The listing builds one solid part. Answer for the finished solid, in the listing's coordinates (mm). Round coordinates to 2 decimals unless told otherwise and drop trailing zeros. Loops run counter-clockwise (first coordinate to the right, second up) from the corner with the lowest first, then second, coordinate; pieces in that order, holes last. Notation, with made-up numbers: M 36,-22.5 L 55,-22.5 A8 cw 55,-16.5 Z; hole C 88,-40 d6. An arc over 180 degrees is marked long. Put each result on its own line as item: value. Start each with the question number.
(1) Straight lines are drawn through the part: line 1 (X direction, y = -20.75, z = 104.9); line 2 (Y direction, x = -20, z = 104.85); line 3 (Y direction, x = 0.5, z = 104.65). For each, find the intervals that lie inside material, in ascending order.
(2) Section C-C, the plane x = 0 is taken. Determine the outline of the cut face in (y, z), then the cut area to 3 significant figures.
(3) Section A-A, the plane z = 104.1 is taken. Determine the outline of the cut face in (x, y).
(4) Determine the mould class of faces 1 (the face through (8, -14, 105.1)), 2 (the face through (0, -8, 104)), 3 (the face through (-1.5, -11.1, 104.4)) for opening direction X: released by +X, released by -X, zero draft, split by the parting line, or undercut.
(5) Section B-B, the plane y = -22.5 is taken. Determine the outline of the cut face in (x, z).
(6) Section D-D, the plane y = -17.25 is taken. Determine the outline of the cut face in (x, z).
```python
from build123d import *

# Parameters (mm, degrees)
SKETCH044_R   = 14.5
SKETCH044_R_2 = 11.5
PAD026_DEPTH  = 1.3
SKETCH045_R   = 2.25
PAD027_DEPTH  = 1.3


with BuildPart() as part:
    # Sketch044 → Pad026 (new body)
    with BuildSketch(Plane.XY):
        Circle(SKETCH044_R)
        Circle(SKETCH044_R_2, mode=Mode.SUBTRACT)
    extrude(amount=PAD026_DEPTH)

    # Sketch045 → Pad027 (join)
    with BuildSketch(Plane.XY):
        with BuildLine():
            Line((-22.781417, 4.431635), (-12, 6.33269))
            Line((-12, 6.33269), (-12, -6.33269))
            Line((-12, -6.33269), (-22.781417, -4.431635))
            ThreePointArc((-22.781417, 4.431635), (-26.5, 0), (-22.781417, -4.431635))
        make_face()
        with Locations((-22, 0)):
            Circle(SKETCH045_R, mode=Mode.SUBTRACT)
    pad027 = extrude(amount=PAD027_DEPTH)

    # Mirrored003: Pad027 across Sketch045 V_Axis
    add(pad027.mirror(Plane(origin=(0, 0, 0), x_dir=(0, 0, 1), z_dir=(1, 0, 0))))


with BuildPart() as part_1:
    # Body026 placement: moved
    add(part.part.moved(Location((0, -22.5, 103.8))))


solid = part_1.part
```
Recorded:
1. line 1: x = -26.15 to -23.41, -20.59 to -11.37, 11.37 to 20.59, 23.41 to 26.15
1. line 2: y = -27.42 to -23.53, -21.47 to -17.58
1. line 3: y = -36.99 to -33.99, -11.01 to -8.01
2. outline: M -37,103.8 L -34,103.8 L -34,105.1 L -37,105.1 Z; M -11,103.8 L -8,103.8 L -8,105.1 L -11,105.1 Z
2. area: 7.80 mm²
3. outline: M -22.78,-26.93 L -13.14,-28.63 A14.5 ccw 13.14,-28.63 L 22.78,-26.93 A4.5 ccw 22.78,-18.07 L 13.14,-16.37 A14.5 ccw -13.14,-16.37 L -22.78,-18.07 A4.5 ccw Z; hole C -22,-22.5 d4.5; hole C 0,-22.5 d23; hole C 22,-22.5 d4.5
4. face 1: zero draft
4. face 2: split by the parting line
4. face 3: undercut
5. outline: M -26.5,103.8 L -24.25,103.8 L -24.25,105.1 L -26.5,105.1 Z; M -19.75,103.8 L -11.5,103.8 L -11.5,105.1 L -19.75,105.1 Z; M 11.5,103.8 L 19.75,103.8 L 19.75,105.1 L 11.5,105.1 Z; M 24.25,103.8 L 26.5,103.8 L 26.5,105.1 L 24.25,105.1 Z
6. outline: M -18.14,103.8 L -10.23,103.8 L -10.23,105.1 L -18.14,105.1 Z; M 10.23,103.8 L 18.14,103.8 L 18.14,105.1 L 10.23,105.1 Z
